Input: part model. Units: mm. Frame: model coordinates. A direction names the side the tool comes from. Round coordinates to 2 decimals unless told otherwise and drop trailing zeros. Loops run counter-clockwise (first coordinate to the right, second up) from the corner with the lowest first, then second, coordinate; pieces in that order, holes last. Notation, with made-up numbers: (34, -5.5) -> (79, -5.5) arc R30 cw to (79, 25.5) -> close; hole circle Ø11 at (67, 77). An arc over 180 degrees is marked (long way). One line per question, with ' | ' between items. Start each with the question number.
Q1. Cut plane B-B on x = 12.25. Return loops of the section in (y, z), and give its area (3 significant figures).
Q2. Contact query for flat-ended pins moving along their axis: P1, Ø1.8, axis at x = 5.89, y = 1.16, coming from the -Z side; P2, Ø1.1, axis at x = 2.09, y = 1.16, coming from the +Z side. Output: stop coordinate, or through.
Q3. Material intervals for L1, parallel to X at y = 2.5, z = 1.55; L2, parallel to X at y = 1, z = 1.3; L3, parallel to X at y = 1.5, z = 1.2, sorted ascending.
Q4. Access query for faces 1 (the face through (4, 11.535, 1)), 2 (the face through (12.468, 5.235, 0.789)). Directions: +Z, -Z, +X, -X, +Y, -Y. A direction counts if a zero-diameter tool reaches every point of the face in a straight line with its end or side. Return the directions, or none.
Q5. Mould query, pull axis Y, two halves, no side actions, for faces 3 (the face through (4, 6, 1.6)), 4 (the face through (6.54, 1.36, 0.79)), 5 (the face through (-4.479, 5.235, 0.789)), 6 (the face through (4, 0.035, 1)). Classes: pulls with the +Y half, pulls with the -Y half, needs draft (parallel to the pull), parting line crosses it, or undercut.
Q6. Cut plane A-A on y = 3.5. Return loops of the section in (x, z).
Q7. Cut plane C-C on z = 0.3. Return loops of the section in (x, y) (3 decimals).
from build123d import *

# Parameters (mm, degrees)
SKETCH2_W           = 23.999949
SKETCH2_H           = 11.5
SKETCH2_R           = 0.675
BOSS_EXTRUDE1_DEPTH = 1.6


with BuildPart() as part:
    # Sketch2 → Boss-Extrude1 (new body)
    with BuildSketch(Plane.XY):
        with Locations((3.994128142, 5.784892068)):
            Rectangle(SKETCH2_W, SKETCH2_H)
        with Locations((2.094154642, 1.159893068)):
            Circle(SKETCH2_R, mode=Mode.SUBTRACT)
        with Locations((5.894154642, 1.159893068)):
            Circle(SKETCH2_R, mode=Mode.SUBTRACT)
        with BuildLine():
            Line((11.294102642, 2.034892068), (11.294102642, 4.034892068))
            ThreePointArc((11.294102642, 4.034892068), (12.494102642, 5.234892068), (13.694102642, 4.034892068))
            Line((13.694102642, 4.034892068), (13.694102642, 2.034892068))
            ThreePointArc((13.694102642, 2.034892068), (12.494102642, 0.834892068), (11.294102642, 2.034892068))
        make_face(mode=Mode.SUBTRACT)
        with BuildLine():
            Line((-3.305846358, 2.034892068), (-3.305846358, 4.034892068))
            ThreePointArc((-3.305846358, 4.034892068), (-4.505846358, 5.234892068), (-5.705846358, 4.034892068))
            Line((-5.705846358, 4.034892068), (-5.705846358, 2.034892068))
            ThreePointArc((-5.705846358, 2.034892068), (-4.505846358, 0.834892068), (-3.305846358, 2.034892068))
        make_face(mode=Mode.SUBTRACT)
    extrude(amount=BOSS_EXTRUDE1_DEPTH)


solid = part.part
Results:
1) outline: (0.03, 0) -> (0.86, 0) -> (0.86, 1.6) -> (0.03, 1.6) -> close; (5.21, 0) -> (11.53, 0) -> (11.53, 1.6) -> (5.21, 1.6) -> close | area: 11.4 mm^2
2) P1: z = 0 | P2: through
3) L1: -8.01 to -5.71, -3.31 to 11.29, 13.69 to 15.99 | L2: -8.01 to -5.11, -3.9 to 1.44, 2.75 to 5.24, 6.55 to 11.89, 13.1 to 15.99 | L3: -8.01 to -5.58, -3.43 to 1.51, 2.68 to 5.31, 6.48 to 11.42, 13.57 to 15.99
4) face 1: +Z, -Z, +X, -X, +Y | face 2: +Z, -Z
5) face 3: needs draft | face 4: undercut | face 5: undercut | face 6: pulls with the -Y half
6) outline: (-8.01, 0) -> (-5.71, 0) -> (-5.71, 1.6) -> (-8.01, 1.6) -> close; (-3.31, 0) -> (11.29, 0) -> (11.29, 1.6) -> (-3.31, 1.6) -> close; (13.69, 0) -> (15.99, 0) -> (15.99, 1.6) -> (13.69, 1.6) -> close
7) outline: (-8.006, 0.035) -> (15.994, 0.035) -> (15.994, 11.535) -> (-8.006, 11.535) -> close; hole (-5.706, 2.035) arc R1.2 ccw to (-3.306, 2.035) -> (-3.306, 4.035) arc R1.2 ccw to (-5.706, 4.035) -> close; hole circle Ø1.35 at (2.094, 1.16); hole circle Ø1.35 at (5.894, 1.16); hole (11.294, 2.035) arc R1.2 ccw to (13.694, 2.035) -> (13.694, 4.035) arc R1.2 ccw to (11.294, 4.035) -> close
